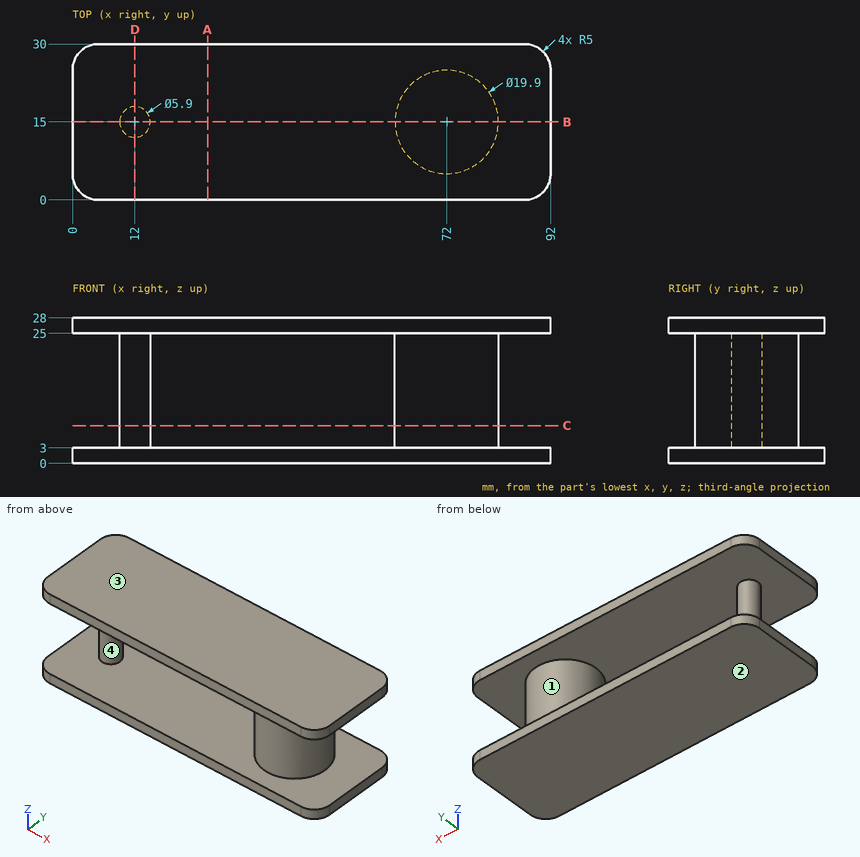
Here's the drawing with two shaded views (mm, measured from the low corner). I have some questions. A direction names the side the tool comes from. Coordinates: 2 decimals unless noted, no trailing zeros. Write each loop counter-clockwise with the first axis right and the second up, starting at its lowest first coordinate (ties: lowest second). Pieces come first, ordered by that corner, then holes.
Item 1: On a 3-axis mill with a long thin cutter (end or side, diameter ignored), from which of +Z, -Z, +X, -X, +Y, -Y can I reach the whole of each face in a straight line? I mean the marked faces 1 and 2. Say none if no direction works.
Item 2: I want a section at B-B on y = 15. Write out the boundary of the cut face in (x, z), and give its area (3 significant figures).
Item 3: I want a section at C-C on z = 7.25. Write out the boundary of the cut face in (x, y), and give its area (3 significant figures).
Item 4: Will these pins go through, and if not, where does the flat tip stop? pin 1 (12 mm diameter, centred on x = 58, z = 13, fed in from +Y); pin 2 (6 mm diameter, centred on y = 8, z = 14.5, fed in from +X); pin 3 (3 mm diameter, centred on y = 10.5, z = 15, fed in from +X).
Item 5: I want a section at D-D on x = 12. Write out the boundary of the cut face in (y, z).
Item 6: If I drill on line 1 (Z direction, x = 11, y = 20); line 2 (X direction, y = 12.5, z = 24.5); line 3 (X direction, y = 13.5, z = 23.25), over which ranges is the centre line in solid material (lowest first)?
Item 7: I want a section at A-A on x = 26. Write out the boundary of the cut face in (y, z), and give its area (3 significant figures).
Item 8: If we mould it in two halves opening along X, with no side actions, what happens to the marked faces 3 and 4? For each: +X half, -X half, draft (parallel to the pull), parting line (faces both ways), or undercut.
Findings below:
1. face 1: none
1. face 2: -Z, +X, -X, +Y, -Y
2. outline: (0, 0) - (92, 0) - (92, 3) - (81.95, 3) - (81.95, 25) - (92, 25) - (92, 28) - (0, 28) - (0, 25) - (9.05, 25) - (9.05, 3) - (0, 3) - close; hole (14.95, 3) - (62.05, 3) - (62.05, 25) - (14.95, 25) - close
2. area: 1,120 mm2
3. outline: circle Ø5.9 at (12, 15); circle Ø19.9 at (72, 15)
3. area: 338 mm2
4. pin 1: stops at y = 20.92
4. pin 2: stops at x = 81.11
4. pin 3: stops at x = 81.49
5. outline: (0, 0) - (30, 0) - (30, 3) - (17.95, 3) - (17.95, 25) - (30, 25) - (30, 28) - (0, 28) - (0, 25) - (12.05, 25) - (12.05, 3) - (0, 3) - close
6. line 1: z = 0 to 3, 25 to 28
6. line 2: x = 10.43 to 13.57, 62.37 to 81.63
6. line 3: x = 9.46 to 14.54, 62.16 to 81.84
7. outline: (0, 0) - (30, 0) - (30, 3) - (0, 3) - close; (0, 25) - (30, 25) - (30, 28) - (0, 28) - close
7. area: 180 mm2
8. face 3: draft
8. face 4: undercut
